```python
from build123d import *

# Parameters (mm, degrees)
BOSS_EXTRU_1_DEPTH      = 60
BOSS_EXTRU_1_DEPTH_BACK = 10
BOSS_EXTRU_2_START      = -50
BOSS_EXTRU_2_DEPTH      = 50
CHANFREIN1_SIZE         = 2


with BuildPart() as part:
    # Esquisse1 → Boss.-Extru.1 (new, two sides: drawn at the far end of the back side and taken through both)
    with BuildSketch(Plane.XY.offset(-BOSS_EXTRU_1_DEPTH_BACK)):
        with BuildLine():
            Line((3.181980515, 2.75), (3.181980515, 3.181980515))
            Line((3.181980515, 3.181980515), (-3.181980515, 3.181980515))
            Line((-3.181980515, 3.181980515), (-3.181980515, -3.181980515))
            Line((-3.181980515, -3.181980515), (3.181980515, -3.181980515))
            Line((3.181980515, -3.181980515), (3.181980515, -2.75))
            Line((3.181980515, -2.75), (9.614442262, -2.75))
            ThreePointArc((9.614442262, -2.75), (-10, 0), (9.614442262, 2.75))
            Line((9.614442262, 2.75), (3.181980515, 2.75))
        make_face()
    extrude(amount=BOSS_EXTRU_1_DEPTH + BOSS_EXTRU_1_DEPTH_BACK)

    # Esquisse3 → Boss.-Extru.2 (add)
    with BuildSketch(Plane.XY.offset(60).offset(BOSS_EXTRU_2_START)):
        with BuildLine():
            Line((5, -8.660254038), (5, -18.660254038))
            Line((5, -18.660254038), (10, -23.660254038))
            Line((10, -23.660254038), (-10, -23.660254038))
            Line((-10, -23.660254038), (-5, -18.660254038))
            Line((-5, -18.660254038), (-5, -8.660254038))
            ThreePointArc((-5, -8.660254038), (0, -10), (5, -8.660254038))
        make_face()
    extrude(amount=BOSS_EXTRU_2_DEPTH)

    # Chanfrein1
    chanfrein1_edges = [part.edges().sort_by_distance(p)[0] for p in [
        (-10, 0, -10),
    ]]
    chamfer(chanfrein1_edges, length=CHANFREIN1_SIZE)


solid = part.part
```
For this review, take the finished solid that the model builds, in its own axes (mm). A direction names the side the tool comes from. Round coordinates to 2 decimals unless told otherwise and drop trailing zeros. Loops run counter-clockwise (first coordinate to the right, second up) from the corner with the lowest first, then second, coordinate; pieces in that order, holes last.
Q1. Add section D-D on z = 37.5. Write out the cut boundary in (x, y), plus the area to 3 significant figures.
Result sheet:
outline: (-10, -23.66) - (10, -23.66) - (5, -18.66) - (5, -8.66) arc R10 ccw to (9.61, -2.75) - (3.18, -2.75) - (3.18, -3.18) - (-3.18, -3.18) - (-3.18, 3.18) - (3.18, 3.18) - (3.18, 2.75) - (9.61, 2.75) arc R10 ccw (long way) to (-5, -8.66) - (-5, -18.66) - close
area: 403 mm2
Q2. To check wall thickness, follow line 1 along Y through (x, z) = (-2.75, 44.5); line 2 along Y through (x, z) = (5.25, 29); line 3 along Y through (x, z) = (9.25, 51.5). State the ranges of each line that lie inside material, in increasing order.
Result sheet:
line 1: y = -23.66 to -3.18, 3.18 to 9.61
line 2: y = -23.66 to -18.91, -8.51 to -2.75, 2.75 to 8.51
line 3: y = -23.66 to -22.91, -3.8 to -2.75, 2.75 to 3.8
Q3. Insertion check: pin 1 Ø0.5 at (y, z) = (3, 16.5) entering from -X; pin 2 Ø3 at (y, z) = (-15, 36) entering from +X; pin 3 Ø1 at (x, z) = (-7, 14) entering from +Y. Each pin has a flat end and moves straight along its axis. Give the tip position at first contact, or say it passes through.
Result sheet:
pin 1: stops at x = -9.61
pin 2: stops at x = 5
pin 3: stops at y = 7.6
Q4. Add section B-B on z = -1. Write out the cut boundary in (x, y), plus the area to 3 significant figures.
Result sheet:
outline: (-3.18, -3.18) - (-3.18, 3.18) - (3.18, 3.18) - (3.18, 2.75) - (9.61, 2.75) arc R10 ccw (long way) to (9.61, -2.75) - (3.18, -2.75) - (3.18, -3.18) - close
area: 237 mm2
Q5. Add section A-A on x = 0. Write out the cut boundary in (y, z), plus the area to 3 significant figures.
Result sheet:
outline: (-23.66, 10) - (-10, 10) - (-10, -8) - (-8, -10) - (-3.18, -10) - (-3.18, 60) - (-23.66, 60) - close; (3.18, -10) - (8, -10) - (10, -8) - (10, 60) - (3.18, 60) - close
area: 1,630 mm2
Q6. Mouldability with a two-part tool opening along X and no side actions: class faces 1 (the face through (0, 3.182, 25)), 2 (the face through (-8.119, -0.326, -9.875)), 3 (the face through (0, -3.182, 25)), 4 (the face through (0, -18, 10)) as +X half, -X half, draft (parallel to the pull), parting line (faces both ways), or undercut.
Result sheet:
face 1: undercut
face 2: parting line
face 3: undercut
face 4: draft
Q7. Machinability: for faces 5 (the face through (6, -2.75, 25)), 6 (the face through (-5, -14, 35)), 7 (the face through (-3.182, 0, 25)), which of the approach directions +Z, -Z, +X, -X, +Y, -Y give a long, thin tool a straight path to every point of the face, cutting with its end or side? Answer none if there is none.
Result sheet:
face 5: +Z, -Z, +X
face 6: +Z, -Z, -X
face 7: +Z, -Z
Q8. Add section C-C on y = 0. Write out the cut boundary in (x, z).
Result sheet:
outline: (-10, -8) - (-8, -10) - (-3.18, -10) - (-3.18, 60) - (-10, 60) - close
